Autodesk Inventor part; units mm, degrees
ref_plane "YZ Plane" through (0, 0, 0) normal (1, 0, 0) x (0, 1, 0)
ref_plane "XZ Plane" through (0, 0, 0) normal (0, 1, 0) x (-1, 0, 0)
ref_plane "XY Plane" through (0, 0, 0) normal (0, 0, 1) x (1, 0, 0)
sketch "Sketch1" plane through (0, 0, 0) normal (0, 0, 1) x (1, 0, 0)
  line L0 (100.775, -66.125) -> (-100.775, -66.125)
  line L1 (-100.775, -66.125) -> (-100.775, 66.125)
  line L2 (-100.775, 66.125) -> (100.775, 66.125)
  line L3 (100.775, 66.125) -> (100.775, -66.125)
  line L4 (100.775, -66.125) -> (-100.775, 66.125) construction
  line L5 (-100.775, -66.125) -> (100.775, 66.125) construction
  point P0 (0, 0)
  dimension "d0" = 201.55
  dimension "d1" = 132.25
extrude "TopPlate" add sketch "Sketch1" along normal blind 5
sketch "Sketch2" plane through (0, 0, 5) normal (0, 0, 1) x (1, 0, 0)
  line L0 (-100.775, -66.125) -> (100.775, -66.125)
  line L1 (-100.775, -66.125) -> (-87.775, -66.125)
  line L2 (-87.775, -66.125) -> (-87.775, -48.125)
  line L3 (-87.775, -48.125) -> (-100.775, -48.125)
  line L4 (-100.775, -48.125) -> (-100.775, -66.125)
  line L5 (100.775, -66.125) -> (100.775, 66.125)
  line L6 (100.775, -66.125) -> (87.775, -66.125)
  line L7 (87.775, -66.125) -> (87.775, -48.125)
  line L8 (87.775, -48.125) -> (100.775, -48.125)
  line L9 (100.775, -48.125) -> (100.775, -66.125)
  line L10 (100.775, 66.125) -> (-100.775, 66.125)
  line L11 (-100.775, 66.125) -> (-87.775, 66.125)
  line L12 (-87.775, 66.125) -> (-87.775, 48.125)
  line L13 (-87.775, 48.125) -> (-100.775, 48.125)
  line L14 (-100.775, 48.125) -> (-100.775, 66.125)
  line L15 (100.775, 66.125) -> (87.775, 66.125)
  line L16 (87.775, 66.125) -> (87.775, 48.125)
  line L17 (87.775, 48.125) -> (100.775, 48.125)
  line L18 (100.775, 48.125) -> (100.775, 66.125)
  line L19 (-100.775, 66.125) -> (-87.775, 48.125)
  line L20 (-87.775, 66.125) -> (-100.775, 48.125)
  line L21 (87.775, 66.125) -> (100.775, 48.125)
  line L22 (100.775, 48.125) -> (100.775, 66.125)
  line L23 (87.775, 48.125) -> (100.775, 66.125)
  line L24 (100.775, -66.125) -> (87.775, -48.125)
  line L25 (100.775, -48.125) -> (87.775, -66.125)
  line L26 (-100.775, -48.125) -> (-87.775, -66.125)
  line L27 (-100.775, 66.125) -> (-100.775, -66.125)
  line L28 (-87.775, -48.125) -> (-100.775, -66.125)
  point P0 (0, 0)
  point P1 (-94.275, -57.125)
  point P2 (-94.275, 57.125)
  point P3 (94.275, 57.125)
  point P4 (94.275, -57.125)
  dimension "d4" = 13
  dimension "d5" = 18
  dimension "d6" = 13
  dimension "d7" = 18
  dimension "d8" = 13
  dimension "d9" = 18
  dimension "d10" = 13
  dimension "d11" = 18
hole "Hole1" at (-94.275, -57.125, 5) at (94.275, 57.125, 5) at (94.275, -57.125, 5) at (-94.275, 57.125, 5) direction (0, 0, -1) diameter 3.4 end through all counterbore diameter 6.5 counterbore depth 3.4
sketch "Sketch34" plane through (0, 0, 5) normal (0, 0, 1) x (1, 0, 0)
  circle A0 centre (43.525, -18.875) radius 6.25
  line L0 (100.775, 66.125) -> (-100.775, 66.125)
  line L1 (-100.775, 66.125) -> (-100.775, -66.125)
  line L2 (-100.775, -66.125) -> (100.775, -66.125)
  point P0 (0, 0)
  point P1 (-125, -13.875)
  point P2 (-125, 66.125)
  point P3 (-125, 66.125)
  point P4 (-65, 66.125)
  point P5 (48.3273, -66.125)
  point P6 (38.7227, -66.125)
  dimension "d166" = 12.5
  dimension "d170" = 144.3
  dimension "d261" = 47.25
extrude "ToggleswitchWithCap1" cut sketch "Sketch34" against normal blind 10
sketch "Sketch38" plane through (0, 0, 5) normal (0, 0, 1) x (1, 0, 0)
  line L0 (68.825, -37.375) -> (82.325, -37.375)
  line L1 (82.325, -37.375) -> (82.325, -57.375)
  line L2 (82.325, -57.375) -> (68.825, -57.375)
  line L3 (68.825, -57.375) -> (68.825, -37.375)
  line L4 (100.775, 66.125) -> (-100.775, 66.125)
  line L5 (-100.775, 66.125) -> (-100.775, -66.125)
  line L6 (-100.775, -66.125) -> (100.775, -66.125)
  point P0 (0, 0)
  dimension "d181" = 13.5
  dimension "d182" = 20
  dimension "d186" = 169.6
  dimension "d266" = 8.75
extrude "OnOffToggle" cut sketch "Sketch38" against normal through all
sketch "Sketch17" plane through (0, 0, 5) normal (0, 0, 1) x (1, 0, 0)
  circle A0 centre (43.525, -47.875) radius 9.5
  line L0 (100.775, 66.125) -> (-100.775, 66.125)
  line L1 (-100.775, 66.125) -> (-100.775, -66.125)
  line L2 (-100.775, -66.125) -> (100.775, -66.125)
  point P0 (0, 0)
  point P1 (-104.4472, 75)
  point P2 (-85.5528, 75)
  point P3 (-125, -57.3222)
  point P4 (-125, -38.4278)
  dimension "d81" = 19
  dimension "d83" = 144.3
  dimension "d223" = 18.25
extrude "KeySwitch" cut sketch "Sketch17" against normal through all
sketch "Sketch18" plane through (0, 0, 5) normal (0, 0, 1) x (1, 0, 0)
  circle A0 centre (-75.775, 46.625) radius 6.25
  line L0 (-100.775, 66.125) -> (-100.775, -66.125)
  line L1 (100.775, 66.125) -> (-100.775, 66.125)
  line L2 (100.775, -66.125) -> (100.775, 66.125)
  point P0 (0, 0)
  point P1 (-11.1695, 75)
  point P2 (1.1695, 75)
  dimension "d86" = 12.5
  dimension "d99" = 19.5
  dimension "d225" = 25
extrude "Toggleswitch1" cut sketch "Sketch18" against normal through all
sketch "Sketch19" plane through (0, 0, 5) normal (0, 0, 1) x (1, 0, 0)
  circle A0 centre (-45.775, 46.625) radius 6.25
  line L0 (100.775, 66.125) -> (-100.775, 66.125)
  line L1 (-100.775, 66.125) -> (-100.775, -66.125)
  line L2 (100.775, -66.125) -> (100.775, 66.125)
  point P0 (0, 0)
  dimension "d89" = 12.5
  dimension "d100" = 19.5
  dimension "d226" = 55
extrude "Toggleswitch2" cut sketch "Sketch19" against normal through all
sketch "Sketch20" plane through (0, 0, 5) normal (0, 0, 1) x (1, 0, 0)
  circle A0 centre (-15.775, 46.625) radius 6.25
  line L0 (100.775, 66.125) -> (-100.775, 66.125)
  line L1 (-100.775, 66.125) -> (-100.775, -66.125)
  line L2 (100.775, -66.125) -> (100.775, 66.125)
  point P0 (0, 0)
  dimension "d92" = 12.5
  dimension "d102" = 19.5
  dimension "d227" = 85
extrude "Toggleswitch3" cut sketch "Sketch20" against normal through all
sketch "Sketch21" plane through (0, 0, 5) normal (0, 0, 1) x (1, 0, 0)
  circle A0 centre (14.225, 46.625) radius 6.25
  line L0 (100.775, 66.125) -> (-100.775, 66.125)
  line L1 (-100.775, 66.125) -> (-100.775, -66.125)
  line L2 (100.775, -66.125) -> (100.775, 66.125)
  point P0 (0, 0)
  dimension "d95" = 12.5
  dimension "d104" = 19.5
  dimension "d228" = 115
extrude "Toggleswitch4" cut sketch "Sketch21" against normal through all
sketch "Sketch22" plane through (0, 0, 5) normal (0, 0, 1) x (1, 0, 0)
  circle A0 centre (-75.775, 6.625) radius 6.1
  line L0 (-100.775, 66.125) -> (-100.775, -66.125)
  line L1 (100.775, 66.125) -> (-100.775, 66.125)
  line L2 (100.775, -66.125) -> (100.775, 66.125)
  point P0 (0, 0)
  dimension "d106" = 12.2
  dimension "d110" = 59.5
  dimension "d229" = 25
extrude "ButtonBlack1" cut sketch "Sketch22" against normal through all
sketch "Sketch23" plane through (0, 0, 5) normal (0, 0, 1) x (1, 0, 0)
  circle A0 centre (-45.775, 6.625) radius 6.1
  line L0 (100.775, 66.125) -> (-100.775, 66.125)
  line L1 (-100.775, 66.125) -> (-100.775, -66.125)
  line L2 (100.775, -66.125) -> (100.775, 66.125)
  point P0 (0, 0)
  dimension "d111" = 12.2
  dimension "d114" = 59.5
  dimension "d230" = 55
extrude "ButtonBlack2" cut sketch "Sketch23" against normal through all
sketch "Sketch24" plane through (0, 0, 5) normal (0, 0, 1) x (1, 0, 0)
  circle A0 centre (-15.775, 6.625) radius 6.1
  line L0 (100.775, 66.125) -> (-100.775, 66.125)
  line L1 (-100.775, 66.125) -> (-100.775, -66.125)
  line L2 (100.775, -66.125) -> (100.775, 66.125)
  point P0 (0, 0)
  dimension "d116" = 12.2
  dimension "d117" = 59.5
  dimension "d231" = 85
extrude "ButtonBlack3" cut sketch "Sketch24" against normal through all
sketch "Sketch25" plane through (0, 0, 5) normal (0, 0, 1) x (1, 0, 0)
  circle A0 centre (14.225, 6.625) radius 6.1
  line L0 (100.775, 66.125) -> (-100.775, 66.125)
  line L1 (-100.775, 66.125) -> (-100.775, -66.125)
  line L2 (100.775, -66.125) -> (100.775, 66.125)
  point P0 (0, 0)
  dimension "d121" = 12.2
  dimension "d205" = 59.5
  dimension "d232" = 115
extrude "ButtonBlack4" cut sketch "Sketch25" against normal through all
sketch "Sketch26" plane through (0, 0, 5) normal (0, 0, 1) x (1, 0, 0)
  circle A0 centre (-75.775, -23.375) radius 6.1
  line L0 (-100.775, 66.125) -> (-100.775, -66.125)
  line L1 (100.775, 66.125) -> (-100.775, 66.125)
  line L2 (100.775, -66.125) -> (100.775, 66.125)
  point P0 (0, 0)
  dimension "d126" = 12.2
  dimension "d128" = 89.5
  dimension "d233" = 25
extrude "ButtonRed1" cut sketch "Sketch26" against normal through all
sketch "Sketch27" plane through (0, 0, 5) normal (0, 0, 1) x (1, 0, 0)
  circle A0 centre (-45.775, -23.375) radius 6.1
  line L0 (100.775, 66.125) -> (-100.775, 66.125)
  line L1 (-100.775, 66.125) -> (-100.775, -66.125)
  line L2 (100.775, -66.125) -> (100.775, 66.125)
  point P0 (0, 0)
  dimension "d131" = 12.2
  dimension "d132" = 89.5
  dimension "d234" = 55
extrude "ButtonRed2" cut sketch "Sketch27" against normal through all
sketch "Sketch28" plane through (0, 0, 5) normal (0, 0, 1) x (1, 0, 0)
  circle A0 centre (-15.775, -23.375) radius 6.1
  line L0 (100.775, 66.125) -> (-100.775, 66.125)
  line L1 (-100.775, 66.125) -> (-100.775, -66.125)
  line L2 (100.775, -66.125) -> (100.775, 66.125)
  point P0 (0, 0)
  dimension "d136" = 12.2
  dimension "d137" = 89.5
  dimension "d235" = 85
extrude "ButtonRed3" cut sketch "Sketch28" against normal through all
sketch "Sketch29" plane through (0, 0, 5) normal (0, 0, 1) x (1, 0, 0)
  circle A0 centre (14.225, -23.375) radius 6.1
  line L0 (100.775, 66.125) -> (-100.775, 66.125)
  line L1 (-100.775, 66.125) -> (-100.775, -66.125)
  line L2 (100.775, -66.125) -> (100.775, 66.125)
  point P0 (0, 0)
  dimension "d141" = 12.2
  dimension "d142" = 89.5
  dimension "d236" = 115
extrude "ButtonRed4" cut sketch "Sketch29" against normal through all
sketch "Sketch39" plane through (0, 0, 5) normal (0, 0, 1) x (1, 0, 0)
  line L0 (-85.775, -40.2112) -> (36.025, -40.2112)
  line L1 (36.025, -40.2112) -> (36.025, -66.125)
  line L2 (36.025, -66.125) -> (-85.775, -66.125)
  line L3 (-85.775, -66.125) -> (-85.775, -40.2112)
  circle A0 centre (43.525, -47.875) radius 9.5
  line L4 (-100.775, -66.125) -> (100.775, -66.125)
  line L5 (-100.775, 66.125) -> (-100.775, -66.125)
  point P0 (0, 0)
  point P1 (36.025, -53.706)
  point P2 (36.025, -42.044)
  point P3 (49.225, -40.275)
  point P4 (50.8905, -53.875)
  dimension "d187" = 7.5
  dimension "d218" = 0
  dimension "d224" = 15
extrude "KeySwitchSideLeft" add sketch "Sketch39" against normal up to surface (5 mm away) contours L0 L1 A0 L2 L3 | L1 A0 picked at (35.6607, -49.2254)
sketch "Sketch40" plane through (0, 0, 5) normal (0, 0, 1) x (1, 0, 0)
  line L0 (51.025, -34.9523) -> (60.7775, -34.9523)
  line L1 (60.7775, -34.9523) -> (60.7775, -58.7516)
  line L2 (60.7775, -58.7516) -> (51.025, -58.7516)
  line L3 (51.025, -58.7516) -> (51.025, -34.9523)
  arc A0 (36.025, -53.706) -> (36.025, -42.044) centre (43.525, -47.875) ccw
  point P0 (0, 0)
  point P1 (51.025, -42.044)
  point P2 (51.025, -53.706)
  dimension "d190" = 7.5
extrude "KeySwitchSideRight" add sketch "Sketch40" against normal up to surface (5 mm away) contours A0 L3
sketch "Sketch44" plane through (0, 0, 5) normal (0, 0, 1) x (1, 0, 0)
  circle A0 centre (-75.775, -52.275) radius 3
  line L0 (-100.775, 66.125) -> (-100.775, -66.125)
  line L1 (100.775, 66.125) -> (-100.775, 66.125)
  point P0 (0, 0)
  dimension "d241" = 6
  dimension "d253" = 25
  dimension "d254" = 118.4
extrude "RotaryEncoder1" cut sketch "Sketch44" against normal through all
sketch "Sketch45" plane through (0, 0, 5) normal (0, 0, 1) x (1, 0, 0)
  circle A0 centre (-45.775, -52.275) radius 3
  line L0 (100.775, 66.125) -> (-100.775, 66.125)
  line L1 (-100.775, 66.125) -> (-100.775, -66.125)
  point P0 (0, 0)
  dimension "d244" = 6
  dimension "d255" = 118.4
  dimension "d256" = 55
extrude "RotaryEncoder2" cut sketch "Sketch45" against normal through all
sketch "Sketch46" plane through (0, 0, 5) normal (0, 0, 1) x (1, 0, 0)
  circle A0 centre (-15.775, -52.275) radius 3
  line L0 (100.775, 66.125) -> (-100.775, 66.125)
  line L1 (-100.775, 66.125) -> (-100.775, -66.125)
  point P0 (0, 0)
  dimension "d247" = 6
  dimension "d257" = 118.4
  dimension "d258" = 85
extrude "RotaryEncoder3" cut sketch "Sketch46" against normal through all
sketch "Sketch47" plane through (0, 0, 5) normal (0, 0, 1) x (1, 0, 0)
  circle A0 centre (14.225, -52.275) radius 3
  line L0 (100.775, 66.125) -> (-100.775, 66.125)
  line L1 (-100.775, 66.125) -> (-100.775, -66.125)
  point P0 (0, 0)
  dimension "d250" = 6
  dimension "d259" = 118.4
  dimension "d260" = 115
extrude "RotaryEncoder4" cut sketch "Sketch47" against normal through all
properties part number "Box Top"
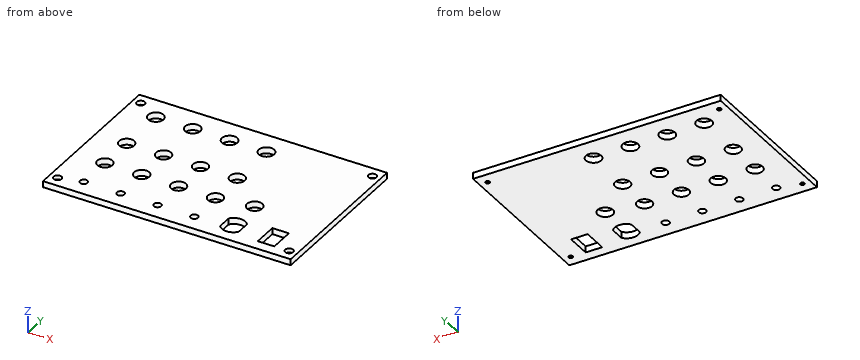
Verification items for the finished model (mm, model axes). Coordinates: 2 decimals unless noted, no trailing zeros. Write each loop counter-clockwise with the first axis right and the second up, starting at its lowest first coordinate (ties: lowest second). Pieces come first, ordered by that corner, then holes. Notation, with made-up numbers: (83, 57.5) - (101, 57.5) arc R22 ccw to (101, 90.5) - close; hole circle Ø7 at (42.5, -11.5). An arc over 180 degrees is marked (long way). One line per question, with ' | ' between items. Start each with the question number.
1. Section check A-A (y = -44). Enter the section's corners in (x, z) (3 decimals), plus the area to 3 significant figures.
2. Gauge pin test, flat ends, axial feed: P1, Ø5, axis at x = 94.275, y = 57.125, coming from the +Z side; P2, Ø7.5, axis at x = -94.275, y = -57.125, coming from the -Z side. Record the tip position at first contact, or that the pin passes through.
3. Material ranges on line 1 along X through (y, z) = (57, 0.9) (3 decimals); line 2 along X through (y, z) = (48, 3.45) (3 decimals); line 3 along Y through (x, z) = (41.5, 2.8) (3 decimals), recorded low to high.
4. Section check B-B (x = -46). Enter the section's corners in (y, z) (3 decimals).
5. Section check C-C (z = 3.1). Count the separate pieces of the cut face and the enclosed holes in it, plus the area to 3 significant figures.
Computed values:
1) outline: (-100.775, 0) - (36.025, 0) - (36.025, 5) - (-100.775, 5) - close; (51.025, 0) - (68.825, 0) - (68.825, 5) - (51.025, 5) - close; (82.325, 0) - (100.775, 0) - (100.775, 5) - (82.325, 5) - close | area: 865 mm²
2) P1: z = 1.6 | P2: z = 0
3) line 1: -100.775 to -95.97, -92.58 to 92.58, 95.97 to 100.775 | line 2: -100.775 to -81.872, -69.678 to -51.872, -39.678 to -21.872, -9.678 to 8.128, 20.322 to 100.775 | line 3: -66.125 to -57.157, -38.593 to -24.788, -12.962 to 66.125
4) outline: (-66.125, 0) - (-55.267, 0) - (-55.267, 5) - (-66.125, 5) - close; (-49.283, 0) - (-29.471, 0) - (-29.471, 5) - (-49.283, 5) - close; (-17.279, 0) - (0.529, 0) - (0.529, 5) - (-17.279, 5) - close; (12.721, 0) - (40.379, 0) - (40.379, 5) - (12.721, 5) - close; (52.871, 0) - (66.125, 0) - (66.125, 5) - (52.871, 5) - close
5) separate pieces: 1 | enclosed holes: 23 | area: 24,300 mm²
